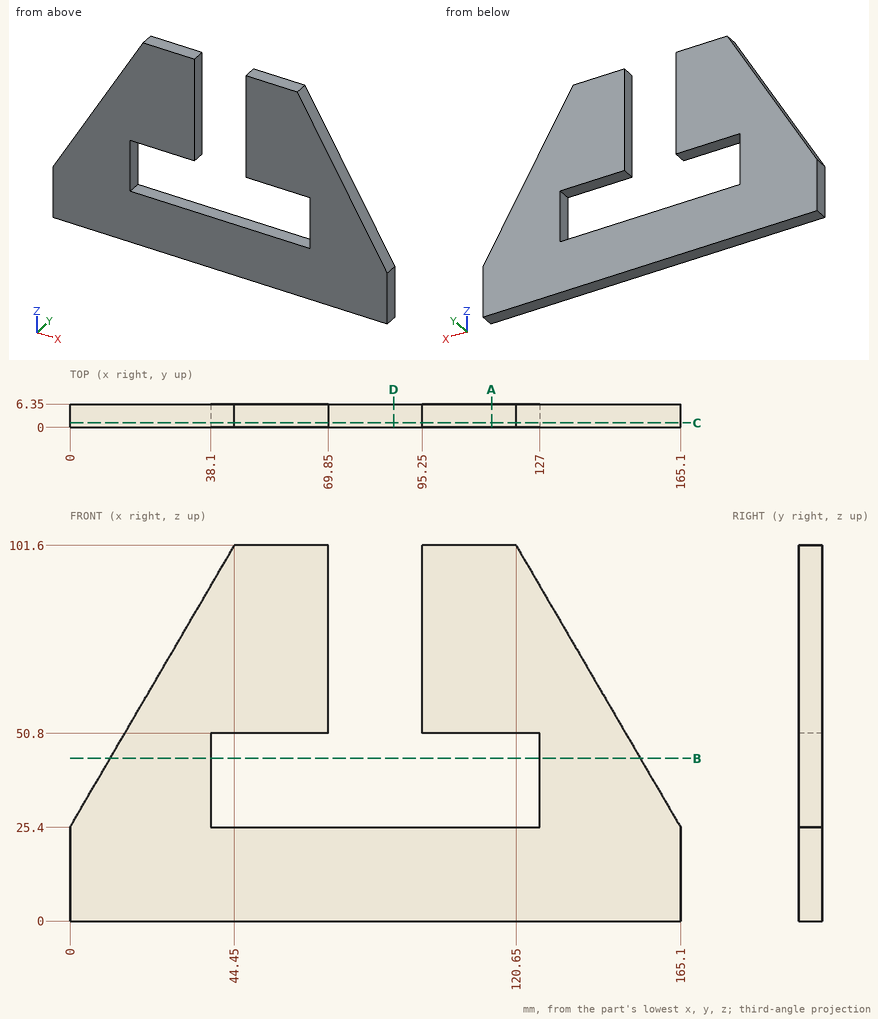
Job drawing, mm, ordinate dimensions from the low corner. One solid piece. Give positions to 0.01 mm unless a question says otherwise; leave off trailing zeros. Order: outer loops, then holes, each group sorted by start corner. A loop starts at its lowest first (then second) coordinate and runs counter-clockwise, first axis right, second up. Notation, with made-up numbers: (-26, -24.75) -> (11, -24.75) arc R28 cw to (11, 11.25) -> close; hole circle Ø9 at (38.25, 51). An arc over 180 degrees is marked (long way). Return JSON: item names as keys, results as strings.
Q1. Saw through at C-C (y = 1.25). Write the cut outline in (x, z), then the cut area to 3 significant figures.
Working result:
{"outline": "(0, 0) -> (165.1, 0) -> (165.1, 25.4) -> (120.65, 101.6) -> (95.25, 101.6) -> (95.25, 50.8) -> (127, 50.8) -> (127, 25.4) -> (38.1, 25.4) -> (38.1, 50.8) -> (69.85, 50.8) -> (69.85, 101.6) -> (44.45, 101.6) -> (0, 25.4) -> close", "area": "9,840 mm²"}
Q2. Drill centre lines: line 1 (Z direction, x = 60, y = 0.5); line 2 (Z direction, x = 84.5, y = 1); line 3 (X direction, y = 2, z = 72). Where is each one in solid material? Low to high.
Working result:
{"line 1": "0 to 25.4, 50.8 to 101.6", "line 2": "0 to 25.4", "line 3": "27.18 to 69.85, 95.25 to 137.92"}
Q3. Flat gauge pins, fed straight in: pin 1 (1.9 mm diameter, centred on y = 2, z = 80.5, fed in from +X); pin 2 (1.5 mm diameter, centred on y = 1.5, z = 28, fed in from -X); pin 3 (1 mm diameter, centred on x = 29, y = 4.5, fed in from +Z). Where does each tip first touch, or does it go through?
Working result:
{"pin 1": "x = 133.51", "pin 2": "x = 1.08", "pin 3": "z = 75.97"}
Q4. Saw through at A-A (x = 114). Write the cut outline in (y, z).
Working result:
{"outline": "(0, 0) -> (6.35, 0) -> (6.35, 25.4) -> (0, 25.4) -> close; (0, 50.8) -> (6.35, 50.8) -> (6.35, 101.6) -> (0, 101.6) -> close"}
Q5. Saw through at B-B (z = 44). Write the cut outline in (x, y), then the cut area to 3 significant figures.
Working result:
{"outline": "(10.85, 0) -> (38.1, 0) -> (38.1, 6.35) -> (10.85, 6.35) -> close; (127, 0) -> (154.25, 0) -> (154.25, 6.35) -> (127, 6.35) -> close", "area": "346 mm²"}
Q6. Saw through at D-D (x = 87.5). Write the cut outline in (y, z), then the cut area to 3 significant figures.
Working result:
{"outline": "(0, 0) -> (6.35, 0) -> (6.35, 25.4) -> (0, 25.4) -> close", "area": "161 mm²"}
